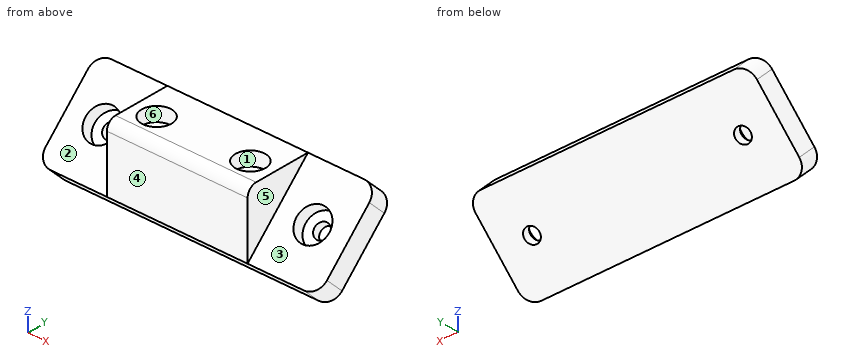
from build123d import *

# Parameters (mm, degrees)
PAD004_DEPTH     = 15
PAD005_DEPTH     = 30
SKETCH009_R      = 3.2
POCKET003_DEPTH  = 3
HOLE_D           = 3.2
HOLE_CBORE_D     = 7
HOLE_CBORE_DEPTH = 3
FILLET_R         = 2
FILLET001_R      = 3


with BuildPart() as part:
    # Sketch007 → Pad004 (new body, symmetric)
    with BuildSketch(Plane.YZ):
        Polygon((0, 0), (-14.142136, -14.142136), (-14.142136, 0), align=None)
    extrude(amount=PAD004_DEPTH, both=True)

    # Sketch008 → Pad005 (join, symmetric)
    with BuildSketch(Plane.YZ):
        Polygon((0, 0), (-14.142136, -14.142136), (-10.606602, -17.67767), (3.535534, -3.535534), align=None)
    extrude(amount=PAD005_DEPTH, both=True)

    # Sketch009 (on Face3 of Pad005) → Pocket003 (cut)
    with BuildSketch(Plane(origin=(0, 0, 0), x_dir=(0, -1, 0), z_dir=(0, 0, 1))):
        with Locations((8, 10)):
            Circle(SKETCH009_R)
        with Locations((8, -10)):
            Circle(SKETCH009_R)
    extrude(amount=-POCKET003_DEPTH, mode=Mode.SUBTRACT)

    # Hole (through all)
    with Locations(Plane(origin=(0, 0, 0), x_dir=(0, -0.707107, -0.707107), z_dir=(0, -0.707107, 0.707107))):
        with Locations((10, 22.5), (10, -22.5)):
            CounterBoreHole(HOLE_D / 2, HOLE_CBORE_D / 2, HOLE_CBORE_DEPTH)

    # Fillet
    fillet_edges = [part.edges().sort_by_distance(p)[0] for p in [
        (0, -14.142136, 0),
    ]]
    fillet(fillet_edges, radius=FILLET_R)

    # Fillet001
    fillet001_edges = [part.edges().sort_by_distance(p)[0] for p in [
        (-30, 1.767767, -1.767767),
        (-30, -12.374369, -15.909903),
        (30, 1.767767, -1.767767),
        (30, -12.374369, -15.909903),
    ]]
    fillet(fillet001_edges, radius=FILLET001_R)


with BuildPart() as part_1:
    # Body002 placement: moved
    add(part.part.moved(Location((0, 55, -10))))


solid = part_1.part
The listing builds one solid part. Answer for the finished solid, in the listing's coordinates (mm). Face numbers are marked on the shaded views. A direction names the side the tool comes from. Coordinates: 2 decimals unless noted, no trailing zeros. Order: outer loops, then holes, each group sorted by start corner. A loop starts at its lowest first (then second) coordinate and runs counter-clockwise, first axis right, second up.
Q1. Which of the six approach directions +Z, -Z, +X, -X, +Y, -Y give full straight-line access (tool end or side, diameter ignored) to the marked faces 1, 2 and 3?
Q2. A cutting plane is placed at B-B, the plane x = -18. Write down the section's boundary in (y, z), and give its area (3 significant figures).
Q3. Given P1, Ø10, axis at x = -3, y = 43.5, coming from the -Z side; P2, Ø4, axis at x = 17.5, z = -15, coming from the -Y side; P3, Ø5, axis at x = -10, y = 47, coming from the +Z side; P4, Ø6, axis at x = -7.5, y = 48.5, coming from the -Z side, each flat-ended and moving along its own axis, determine where each tip first touches the part or whether it passes through.
Q4. Consider line 1 (X direction, y = 47, z = -12.25); line 2 (X direction, y = 47.5, z = -19.75); line 3 (X direction, y = 43.25, z = -20.25). Determine where each line is inside the solid, lowest interval first.
Q5. A cutting plane is placed at A-A, the plane x = 10. Write down the section's boundary in (y, z).
Q6. For a pull along Y with two mould halves and no side action, classify the marked faces 4, 5 and 6 as pulls with the +Y half, pulls with the -Y half, needs draft (parallel to the pull), parting line crosses it, or undercut.
Answers follow:
1. face 1: +Z
1. face 2: +Z, -X, -Y
1. face 3: +Z, +X, -Y
2. outline: (40.86, -24.14) - (44.39, -27.68) - (58.54, -13.54) - (55, -10) - close
2. area: 100 mm2
3. P1: stops at z = -27.68
3. P2: stops at y = 48
3. P3: stops at z = -13
3. P4: stops at z = -26.57
4. line 1: x = -15 to -13.2, -6.8 to 6.8, 13.2 to 15
4. line 2: x = -30 to -25.22, -19.78 to 19.78, 25.22 to 30
4. line 3: x = -15 to 15
5. outline: (40.86, -24.14) - (44.39, -27.68) - (58.54, -13.54) - (55, -10) - (50.2, -10) - (50.2, -13) - (43.8, -13) - (43.8, -10) - (42.86, -10) arc R2 ccw to (40.86, -12) - close
6. face 4: pulls with the -Y half
6. face 5: needs draft
6. face 6: undercut
